from build123d import *

# Parameters (mm, degrees)
SKETCH2_R           = 1.5
CUT_EXTRUDE1_DEPTH  = 6
SKETCH3_R           = 1.25
BOSS_EXTRUDE1_DEPTH = 20


with BuildPart() as part:
    # Sketch1 → Revolve2 (revolve)
    with BuildSketch(Plane.XY, mode=Mode.PRIVATE) as revolve2_sk:
        Polygon((14.4, -45.024704817), (14.4, -20.024704817), (12.4, -18.024704817), (4.5, -18.024704817), (4.5, -16.024704817), (0, -16.024704817), (0, -70.024704817), (2, -70.024704817), (2, -58.36883633), (3.9, -58.36883633), (3.9, -55.824704817), (2.9, -54.824704817), (2, -54.824704817), (2, -54.024704817), (12.4, -54.024704817), align=None)
    revolve(revolve2_sk.sketch.rotate(Axis((0, 0, 0), (0, -1, 0)), 90), axis=Axis((0, 0, 0), (0, -1, 0)))

    # Sketch2 → Cut-Extrude1 (cut)
    with BuildSketch(Plane.XZ.offset(54.024704817)):
        with Locations(Location((6.717514421, 6.717514421, 0), (0, 0, 270))):
            Circle(SKETCH2_R)
        with Locations(Location((5.656854249, -5.656854249, 0), (0, 0, 270))):
            Circle(SKETCH2_R)
        with Locations(Location((-6.717514421, -6.717514421, 0), (0, 0, 270))):
            Circle(SKETCH2_R)
        with Locations(Location((-5.656854249, 5.656854249, 0), (0, 0, 270))):
            Circle(SKETCH2_R)
    extrude(amount=-CUT_EXTRUDE1_DEPTH, mode=Mode.SUBTRACT)

    # Sketch3 → Boss-Extrude1 (add)
    with BuildSketch(Plane.XY.offset(10)):
        with Locations(Location((0, -52.024704817, 0), (0, 0, 224.284221248))):
            Circle(SKETCH3_R)
        with Locations(Location((3.75, -52.024704817, 0), (0, 0, 235.024751842))):
            Circle(SKETCH3_R)
        with Locations(Location((-3.75, -52.024704817, 0), (0, 0, 235.074308892))):
            Circle(SKETCH3_R)
    extrude(amount=BOSS_EXTRUDE1_DEPTH)


solid = part.part
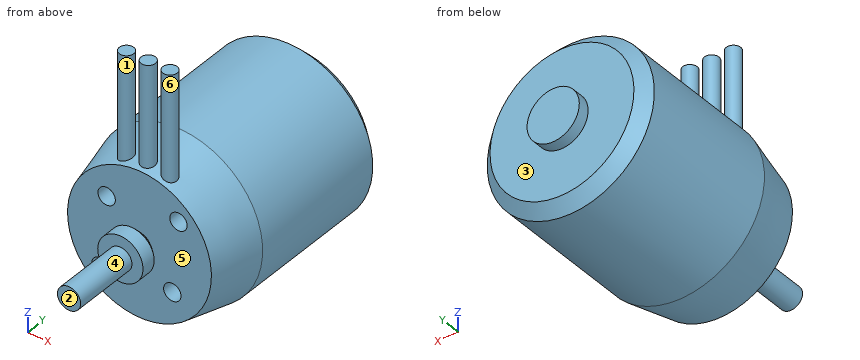
Can you work these out from the model? Positions are in its coordinate system, mm. Face numbers are marked on the shaded views. A direction names the side the tool comes from. Coordinates: 2 decimals unless noted, no trailing zeros. Order: outer loops, then holes, each group sorted by start corner. A loop starts at its lowest first (then second) coordinate and runs counter-clockwise, first axis right, second up. Notation, with made-up numbers: (15, 42) - (37, 42) arc R26 cw to (37, 66) - close; hole circle Ø8 at (53, 61.5). An arc over 180 degrees is marked (long way). Answer as a JSON object with one key per item and string values. Group by question number.
Q1. Will these pins go through, and if not, where does the flat tip stop? P1, Ø5, axis at y = -24.5, z = -6.5, coming from the -X side; P2, Ø1.8, axis at x = 5.66, z = -5.66, coming from the +Y side; P3, Ø1.5, axis at x = -5.5, z = 5, coming from the -Y side; P4, Ø8, axis at y = -46.5, z = 20.5, coming from the +X side.
Q2. Imagine slicing it at D-D (z = 24). Please give me the cut outline in (x, y).
Q3. Imagine slicing it at A-A (z = 0). Please give me the cut outline in (x, y).
Q4. On a 3-axis mill with a long thin cutter (end or side, diameter ignored), from which of +Z, -Z, +X, -X, +Y, -Y can I reach the whole of each face in a straight line? I mean the marked faces 1, 2 and 3. Say none if no direction works.
Q5. Imagine slicing it at C-C (y = -27.5). Please give me the cut outline in (x, z), and give its area (3 significant figures).
Q6. I need wall thicknesses on line 1 (Y direction, x = 1.5, z = -1.5); line 2 (Y direction, x = 5.5, z = 10); line 3 (X direction, y = -51, z = 7). Which ranges of each line are inside material? Lowest first, please. Write a range as from..to.
Q7. We'd pull the mould along X, two halves only. Please class the marked faces 4, 5 and 6: +X half, -X half, draft (parallel to the pull), parting line (faces both ways), or undercut.
Determined:
{
 "1": {"P1": "stops at x = -13.83", "P2": "stops at y = -18.02", "P3": "stops at y = -48.02", "P4": "passes through"},
 "2": {"outline": "circle Ø2.5 at (-3.75, -52.02); circle Ø2.5 at (0, -52.02); circle Ø2.5 at (3.75, -52.02)"},
 "3": {"outline": "(-14.4, -45.02) - (-12.4, -54.02) - (-2, -54.02) - (-2, -54.82) - (-2.9, -54.82) - (-3.9, -55.82) - (-3.9, -58.37) - (-2, -58.37) - (-2, -70.02) - (2, -70.02) - (2, -58.37) - (3.9, -58.37) - (3.9, -55.82) - (2.9, -54.82) - (2, -54.82) - (2, -54.02) - (12.4, -54.02) - (14.4, -45.02) - (14.4, -20.02) - (12.4, -18.02) - (4.5, -18.02) - (4.5, -16.02) - (-4.5, -16.02) - (-4.5, -18.02) - (-12.4, -18.02) - (-14.4, -20.02) - close"},
 "4": {"face 1": "+Z", "face 2": "+Z, -Z, +X, -X, -Y", "face 3": "+Y"},
 "5": {"outline": "circle Ø28.8 at (0, 0)", "area": "651 mm2"},
 "6": {"line 1": "y = -58.37..-54.82, -54.02..-16.02", "line 2": "y = -54.02..-18.02", "line 3": "x = -11.04..-6.32, -4.99..5.24, 8.19..11.04"},
 "7": {"face 4": "parting line", "face 5": "draft", "face 6": "undercut"}
}
